```python
from build123d import *

# Parameters (mm, degrees)
CUT_EXTRUDE1_DEPTH        = 1.04
SKETCH4_R                 = 1.5
LARGO_Y_ANCHO_ROSCA_DEPTH = 6
FILLET1_R                 = 0.1
CHAMFER1_SIZE             = 0.2805


with BuildPart() as part:
    # Sketch1 → Revolve1 (revolve)
    with BuildSketch(Plane(origin=(0, 0, 0), x_dir=(-1, 0, 0), z_dir=(0, 0, -1)), mode=Mode.PRIVATE) as revolve1_sk:
        with BuildLine():
            Line((-1.65, 2.75), (-1.65, 0))
            Line((-1.65, 0), (0, 0))
            Line((0, 0), (0, 1.425))
            ThreePointArc((0, 1.425), (-0.542530893, 2.176130767), (-1.27, 2.75))
            Line((-1.27, 2.75), (-1.65, 2.75))
        make_face()
    revolve(revolve1_sk.sketch.rotate(Axis((1.65, 0, 0), (-1, 0, 0)), 270), axis=Axis((1.65, 0, 0), (-1, 0, 0)))

    # Sketch2 → Cut-Extrude1 (cut)
    with BuildSketch(Plane.ZY):
        Polygon((-1, 0.577350269), (-1, -0.577350269), (0, -1.154700538), (1, -0.577350269), (1, 0.577350269), (0, 1.154700538), align=None)
    extrude(amount=-CUT_EXTRUDE1_DEPTH, mode=Mode.SUBTRACT)

    # Sketch3 → Cut-Revolve1 (revolve, cut)
    with BuildSketch(Plane.XY, mode=Mode.PRIVATE) as cut_revolve1_sk:
        Polygon((1.04, 1), (1.04, 0), (1.617350269, 0), align=None)
    revolve(cut_revolve1_sk.sketch.rotate(Axis((1.04, 0, 0), (1, 0, 0)), 90), axis=Axis((1.04, 0, 0), (1, 0, 0)), mode=Mode.SUBTRACT)

    # Sketch4 → Largo y Ancho rosca (add)
    with BuildSketch(Plane(origin=(1.65, 0, 0), x_dir=(0, 0, -1), z_dir=(1, 0, 0))):
        Circle(SKETCH4_R)
    extrude(amount=LARGO_Y_ANCHO_ROSCA_DEPTH)

    # Fillet1
    fillet1_edges = [part.edges().sort_by_distance(p)[0] for p in [
        (1.65, 0, 1.5),
    ]]
    fillet(fillet1_edges, radius=FILLET1_R)

    # Chamfer1
    chamfer1_edges = [part.edges().sort_by_distance(p)[0] for p in [
        (7.65, 0, 1.5),
    ]]
    chamfer(chamfer1_edges, length=CHAMFER1_SIZE)


solid = part.part
```
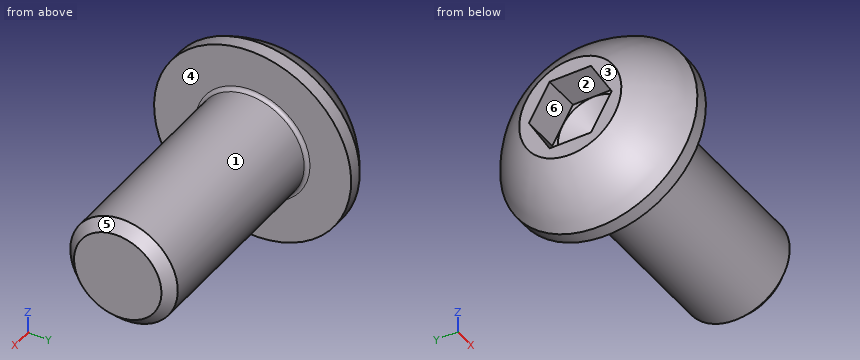
Source: CAD feature listing. Evaluate the final solid. Frame: model axes, mm. Face numbers are marked on the shaded views. A direction names the side the tool comes from. Give positions to 0.01 mm unless a question says otherwise; leave off trailing zeros. Order: outer loops, then holes, each group sorted by start corner. A loop starts at its lowest first (then second) coordinate and runs counter-clockwise, first axis right, second up. Notation, with made-up numbers: (-28.5, 50) -> (16.5, 50) arc R9 ccw to (16.5, 64) -> close; hole circle Ø11 at (25, 1.25). An arc over 180 degrees is marked (long way). Use a Markdown table: item, result.
Q1. Section A-A (x = 3.5). Return the cut outline in (y, z), and give its area (3 significant figures).
A:
| item | result |
|---|---|
| outline | circle Ø3 at (0, 0) |
| area | 7.07 mm^2 |
Q2. Material intervals for line 1 (Z direction, x = 0.5, y = -0.25); line 2 (Y direction, x = 3.25, z = 0), sorted ascending. Write a range as [from, to].
A:
| item | result |
|---|---|
| line 1 | [-2.12, -1], [1, 2.12] |
| line 2 | [-1.5, 1.5] |
Q3. Pull-direction query (Z, two-part tool) for the marked faces 4, 5 and 6; classes: +Z half, -Z half, draft (parallel to the pull), parting line (faces both ways), or undercut.
A:
| item | result |
|---|---|
| face 4 | draft |
| face 5 | parting line |
| face 6 | undercut |
Q4. Access query for the marked faces 1, 2 and 3. Directions: +Z, -Z, +X, -X, +Y, -Y. A direction counts if a zero-diameter tool reaches every point of the face in a straight line with its end or side. Return the directions, or none.
A:
| item | result |
|---|---|
| face 1 | +X |
| face 2 | -X |
| face 3 | +Z, -Z, -X, +Y, -Y |
Q5. First-contact query: P1, Ø1, axis at x = 3, z = 0, coming from the +Y side; P2, Ø1, axis at x = 1.5, z = -1, coming from the +Y side; P3, Ø3, axis at x = 2.5, y = 2, coming from the -Z side. Flat tips, straight axial feed; report the tip coordinate or a pass-through.
A:
| item | result |
|---|---|
| P1 | y = 1.5 |
| P2 | y = 2.7 |
| P3 | z = -2.64 |
